Autodesk Inventor part; units mm, degrees
ref_plane "YZ Plane" through (0, 0, 0) normal (1, 0, 0) x (0, 1, 0)
ref_plane "XZ Plane" through (0, 0, 0) normal (0, 1, 0) x (-1, 0, 0)
ref_plane "XY Plane" through (0, 0, 0) normal (0, 0, 1) x (1, 0, 0)
sketch "Sketch1" plane through (0, 0, 0) normal (0, 1, 0) x (-1, 0, 0)
  circle A0 centre (0, 0) radius 4
  circle A1 centre (-20, 0) radius 2
  circle A2 centre (20, 0) radius 2
  circle A3 centre (0, 0) radius 7.5
  line L0 (0, 0) -> (20, 0) construction
  circle A4 centre (0, 0) radius 3.9303 construction
  line L1 (0, 0) -> (39.9, 0) construction
  circle A5 centre (39.9, 0) radius 9.875
  line L2 (-20, 0) -> (-25, 0)
  line L3 (-25, 0) -> (-25, 17.5)
  line L4 (-25, 17.5) -> (60, 17.5)
  line L5 (60, 17.5) -> (60, -17.5)
  line L6 (60, -17.5) -> (-25, -17.5)
  line L7 (-25, -17.5) -> (-25, 17.5)
  dimension "d0" = 8
  dimension "d1" = 39.9
  dimension "d2" = 19.75
  dimension "d3" = 5
  dimension "d4" = 17.5
  dimension "d5" = 85
  dimension "d6" = 35
extrude "Extrusion1" add sketch "Sketch1" along normal blind 10 contours L3 L4 L5 L6 L7
fillet "Fillet1" radius 16 2 edges at (-60, 5, -17.5) (-60, 5, 17.5)
properties part number "Bear_fix"
For this review, take the finished solid that the model builds, in its own axes (mm). Coordinates: 2 decimals unless noted, no trailing zeros. Order: outer loops, then holes, each group sorted by start corner. A loop starts at its lowest first (then second) coordinate and runs counter-clockwise, first axis right, second up. Notation, with made-up numbers: (-25, 60) - (1, 60) arc R22 cw to (1, 93) - close; hole circle Ø7 at (10.25, -13). An arc over 180 degrees is marked (long way). Answer as CSV lines item,"result". Start each with the question number.
1) Insertion check: P1, Ø12, axis at x = -39.9, z = 0, coming from the -Y side; P2, Ø1.5, axis at y = 4.5, z = 8, coming from the -X side; P3, Ø3, axis at x = -51.5, y = 7.5, coming from the +Z side. Each pin has a flat end and moves straight along its axis. Give the tip position at first contact, or say it passes through.
2) To check wall thickness, follow line 1 along Z through (x, y) = (-20, 6.5); line 2 along Z through (x, y) = (0, 7.5); line 3 along X through (y, z) = (3, -1.5). State the ranges of each line that lie inside material, in increasing order. Write a range as [from, to].
3) Add section B-B (x = 20). State the section outline as (y, z) points, then the cut area to 3 significant figures.
4) Add section C-C (y = 3.75). State the section outline as (x, z) points (3 decimals).
5) Add section A-A (z = 0). State the section outline as (x, y) points (3 decimals).
6) Add section D-D (z = 5). State the section outline as (x, y) points.
7) Draft analysis for pull direction Z (two halves, no side actions). For faces 1 (the flat face through (25, 5, 0)), 2 (the cylindrical face through (-55.189, 5.07, -12.937)), 3 (the cylindrical face through (-37.76, 4.93, 9.64)), state which applies: +Z half, -Z half, draft (parallel to the pull), parting line (faces both ways), or undercut.
Result:
1,P1,"through"
1,P2,"x = -58.93"
1,P3,"z = 16.33"
2,line 1,"[-17.5, -2], [2, 17.5]"
2,line 2,"[-17.5, -7.5], [7.5, 17.5]"
2,line 3,"[-60, -49.66], [-30.14, -21.32], [-18.68, -7.35], [7.35, 18.68], [21.32, 25]"
3,outline,"(0, -17.5) - (10, -17.5) - (10, -2) - (0, -2) - close; (0, 2) - (10, 2) - (10, 17.5) - (0, 17.5) - close"
3,area,"310 mm^2"
4,outline,"(-60, -1.5) arc R16 ccw to (-44, -17.5) - (25, -17.5) - (25, 17.5) - (-44, 17.5) arc R16 ccw to (-60, 1.5) - close; hole circle Ø19.75 at (-39.9, 0); hole circle Ø4 at (-20, 0); hole circle Ø15 at (0, 0); hole circle Ø4 at (20, 0)"
5,outline,"(-60, 0) - (-49.775, 0) - (-49.775, 10) - (-60, 10) - close; (-30.025, 0) - (-22, 0) - (-22, 10) - (-30.025, 10) - close; (-18, 0) - (-7.5, 0) - (-7.5, 10) - (-18, 10) - close; (7.5, 0) - (18, 0) - (18, 10) - (7.5, 10) - close; (22, 0) - (25, 0) - (25, 10) - (22, 10) - close"
6,outline,"(-59.61, 0) - (-48.42, 0) - (-48.42, 10) - (-59.61, 10) - close; (-31.38, 0) - (-5.59, 0) - (-5.59, 10) - (-31.38, 10) - close; (5.59, 0) - (25, 0) - (25, 10) - (5.59, 10) - close"
7,face 1,"draft"
7,face 2,"-Z half"
7,face 3,"undercut"
